```python
from build123d import *

# Parameters (mm, degrees)
BOSS_EXTRUDE1_DEPTH = 14.2748
SKETCH2_R           = 6.35
SKETCH2_R_2         = 2.4892
BOSS_EXTRUDE2_DEPTH = 7.9502


with BuildPart() as part:
    # Sketch1 → Boss-Extrude1 (new, symmetric)
    with BuildSketch(Plane.XY):
        Polygon((0, 7.332348419), (-6.35, 3.666174209), (-6.35, -3.666174209), (0, -7.332348419), (6.35, -3.666174209), (6.35, 3.666174209), align=None)
    extrude(amount=BOSS_EXTRUDE1_DEPTH, both=True)

    # Sketch2 → Boss-Extrude2 (add)
    with BuildSketch(Plane.XY.offset(14.2748)):
        Circle(SKETCH2_R)
        Circle(SKETCH2_R_2, mode=Mode.SUBTRACT)
    boss_extrude2 = extrude(amount=BOSS_EXTRUDE2_DEPTH)

    # Mirror1: Boss-Extrude2 across plane
    add(boss_extrude2.mirror(Plane.XY))


solid = part.part
```
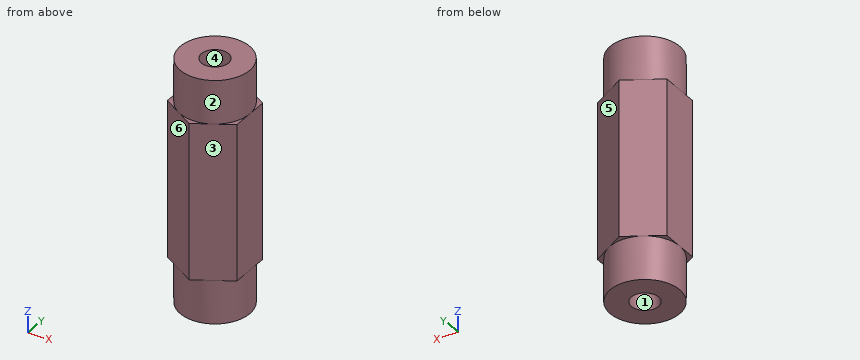
Build history of the part. All positions in model axes, mm. Face numbers are marked on the shaded views. A direction names the side the tool comes from. Give positions to 0.01 mm unless a question says otherwise; leave off trailing zeros. Loops run counter-clockwise (first coordinate to the right, second up) from the corner with the lowest first, then second, coordinate; pieces in that order, holes last.
Item 1: Flat gauge pins, fed straight in: pin 1 (1.5 mm diameter, centred on x = 0.5, z = -7.5, fed in from -Y); pin 2 (1 mm diameter, centred on x = -2, z = 16, fed in from -Y); pin 3 (3 mm diameter, centred on x = 5, z = -1.5, fed in from +Y). Where does each tip first touch, or does it go through?
Answers follow:
pin 1: stops at y = -7.33
pin 2: stops at y = -6.17
pin 3: stops at y = 5.31
Item 2: Slice it at C-C, the plane z = -4.5. List the corners of the cut face in (x, y), and give its area (3 significant figures).
Answers follow:
outline: (-6.35, -3.67) - (0, -7.33) - (6.35, -3.67) - (6.35, 3.67) - (0, 7.33) - (-6.35, 3.67) - close
area: 140 mm2
Item 3: Slice it at D-D, the plane y = 3.25. List the corners of the cut face in (x, z) (3 decimals).
Answers follow:
outline: (-6.35, -14.275) - (-5.455, -14.275) - (-5.455, -22.225) - (5.455, -22.225) - (5.455, -14.275) - (6.35, -14.275) - (6.35, 14.275) - (5.455, 14.275) - (5.455, 22.225) - (-5.455, 22.225) - (-5.455, 14.275) - (-6.35, 14.275) - close
Item 4: Slice it at A-A, the plane y = -1.25. List the corners of the cut face in (x, z) (3 decimals), and give its area (3 significant figures).
Answers follow:
outline: (-6.35, -14.275) - (-6.226, -14.275) - (-6.226, -22.225) - (-2.153, -22.225) - (-2.153, -14.275) - (2.153, -14.275) - (2.153, -22.225) - (6.226, -22.225) - (6.226, -14.275) - (6.35, -14.275) - (6.35, 14.275) - (6.226, 14.275) - (6.226, 22.225) - (2.153, 22.225) - (2.153, 14.275) - (-2.153, 14.275) - (-2.153, 22.225) - (-6.226, 22.225) - (-6.226, 14.275) - (-6.35, 14.275) - close
area: 492 mm2
Item 5: Which spindle directions (+Z, -Z, +X, -X, +Y, -Y) get a long thin tool onto all of the face, cutting with end or side? Do the marked faces 1, 2 and 3. Say none if no direction does.
Answers follow:
face 1: -Z
face 2: +Z
face 3: +Z, -Z, +X, -Y
Item 6: Pull direction X, two halves, no side cores. Call the marked faces 4, 5 and 6: released by +X, released by -X, zero draft, split by the parting line, or undercut.
Answers follow:
face 4: undercut
face 5: released by +X
face 6: released by -X
Item 7: Drill centre lines: line 1 (Y direction, x = 0, z = 19.5); line 2 (Z direction, x = 0.25, y = 6.5); line 3 (X direction, y = 0.75, z = -17). Where is each one in solid material? Low to high.
Answers follow:
line 1: y = -6.35 to -2.49, 2.49 to 6.35
line 2: z = -14.27 to 14.27
line 3: x = -6.31 to -2.37, 2.37 to 6.31
Item 8: Slice it at B-B, the plane x = -4.5. List the corners of the cut face in (y, z) (3 decimals).
Answers follow:
outline: (-4.734, -14.275) - (-4.48, -14.275) - (-4.48, -22.225) - (4.48, -22.225) - (4.48, -14.275) - (4.734, -14.275) - (4.734, 14.275) - (4.48, 14.275) - (4.48, 22.225) - (-4.48, 22.225) - (-4.48, 14.275) - (-4.734, 14.275) - close
